Autodesk Inventor part; units mm, degrees
ref_plane "YZ Plane" through (0, 0, 0) normal (1, 0, 0) x (0, 1, 0)
ref_plane "XZ Plane" through (0, 0, 0) normal (0, 1, 0) x (-1, 0, 0)
ref_plane "XY Plane" through (0, 0, 0) normal (0, 0, 1) x (1, 0, 0)
sketch "Schizzo1" plane through (0, 0, 0) normal (0, 1, 0) x (-1, 0, 0)
  line L0 (10.5, 8) -> (-10.5, 8)
  line L1 (-10.5, 8) -> (-10.5, -8)
  line L2 (-10.5, -8) -> (10.5, -8)
  line L3 (10.5, -8) -> (10.5, 8)
  line L4 (10.5, 8) -> (-10.5, -8) construction
  line L5 (-10.5, 8) -> (10.5, -8) construction
  point P0 (0, 0)
  point P1 (0, 0)
  point P2 (0, 0)
  dimension "d0" = 16
  dimension "d1" = 21
extrude "Estrusione1" add sketch "Schizzo1" along normal blind 1.5
sketch "Schizzo2" plane through (0, 1.5, 0) normal (0, 1, 0) x (1, 0, 0)
  line L0 (10.5, 8) -> (-10.5, 8)
  line L1 (-10.5, 8) -> (-8, 8)
  line L2 (-8, 8) -> (-8, 5.5)
  line L3 (10.5, 8) -> (8, 8)
  line L4 (8, 8) -> (8, 5.5)
  point P0 (0, 0)
  dimension "d16" = 2.5
  dimension "d17" = 2.5
  dimension "d18" = 2.5
  dimension "d19" = 2.5
hole "Foro1" at (-8, 1.5, -5.5) at (8, 1.5, -5.5) direction (0, -1, 0) diameter 3.4 depth 1.5 tip angle 118
sketch "Schizzo4" plane through (0, 1.5, 0) normal (0, 1, 0) x (1, 0, 0)
  line L0 (10, -5.5) -> (-10, -5.5)
  line L1 (-10, -5.5) -> (-10, -8)
  line L2 (-10, -8) -> (10, -8)
  line L3 (10, -8) -> (10, -5.5)
  line L4 (10, -5.5) -> (-10, -8) construction
  line L5 (-10, -5.5) -> (10, -8) construction
  line L6 (-10.5, -8) -> (10.5, -8)
  point P0 (0, 0)
  point P1 (0, -6.75)
  point P2 (0, -8)
  dimension "d45" = 20
  dimension "d46" = 2.5
extrude "Estrusione2" add sketch "Schizzo4" along normal blind 2.5
sketch "Schizzo6" plane through (0, 4, 0) normal (0, 1, 0) x (1, 0, 0)
  line L0 (-8.75, -6.75) -> (-6.25, -6.75)
  line L1 (-9.05, -7.05) -> (-9.05, -6.45)
  line L2 (-9.05, -6.45) -> (-8.45, -6.45)
  line L3 (-8.45, -6.45) -> (-8.45, -7.05)
  line L4 (-8.45, -7.05) -> (-9.05, -7.05)
  line L5 (-6.25, -6.75) -> (-3.75, -6.75)
  line L6 (-6.55, -7.05) -> (-6.55, -6.45)
  line L7 (-6.55, -6.45) -> (-5.95, -6.45)
  line L8 (-5.95, -6.45) -> (-5.95, -7.05)
  line L9 (-5.95, -7.05) -> (-6.55, -7.05)
  line L10 (-3.75, -6.75) -> (-1.25, -6.75)
  line L11 (-4.05, -7.05) -> (-4.05, -6.45)
  line L12 (-4.05, -6.45) -> (-3.45, -6.45)
  line L13 (-3.45, -6.45) -> (-3.45, -7.05)
  line L14 (-3.45, -7.05) -> (-4.05, -7.05)
  line L15 (-1.25, -6.75) -> (1.25, -6.75)
  line L16 (-1.55, -7.05) -> (-1.55, -6.45)
  line L17 (-1.55, -6.45) -> (-0.95, -6.45)
  line L18 (-0.95, -6.45) -> (-0.95, -7.05)
  line L19 (-0.95, -7.05) -> (-1.55, -7.05)
  line L20 (1.25, -6.75) -> (3.75, -6.75)
  line L21 (0.95, -7.05) -> (0.95, -6.45)
  line L22 (0.95, -6.45) -> (1.55, -6.45)
  line L23 (1.55, -6.45) -> (1.55, -7.05)
  line L24 (1.55, -7.05) -> (0.95, -7.05)
  line L25 (3.75, -6.75) -> (6.25, -6.75)
  line L26 (3.45, -7.05) -> (3.45, -6.45)
  line L27 (3.45, -6.45) -> (4.05, -6.45)
  line L28 (4.05, -6.45) -> (4.05, -7.05)
  line L29 (4.05, -7.05) -> (3.45, -7.05)
  line L30 (6.25, -6.75) -> (8.75, -6.75)
  line L31 (5.95, -7.05) -> (5.95, -6.45)
  line L32 (5.95, -6.45) -> (6.55, -6.45)
  line L33 (6.55, -6.45) -> (6.55, -7.05)
  line L34 (6.55, -7.05) -> (5.95, -7.05)
  line L35 (8.45, -7.05) -> (8.45, -6.45)
  line L36 (8.45, -6.45) -> (9.05, -6.45)
  line L37 (9.05, -6.45) -> (9.05, -7.05)
  line L38 (9.05, -7.05) -> (8.45, -7.05)
  line L39 (-8.75, -6.75) -> (-10, -6.75)
  line L40 (-10, -8) -> (10, -8)
  line L41 (-10, -8) -> (-10, -6.75)
  line L42 (-10, -8) -> (-8.75, -8) construction
  point P0 (0, 0)
  dimension "d47" = 2.5
  dimension "d48" = 0.6
  dimension "d49" = 2.5
  dimension "d50" = 0.6
  dimension "d51" = 2.5
  dimension "d52" = 0.6
  dimension "d53" = 2.5
  dimension "d54" = 0.6
  dimension "d55" = 2.5
  dimension "d56" = 0.6
  dimension "d57" = 2.5
  dimension "d58" = 0.6
  dimension "d59" = 2.5
  dimension "d60" = 0.6
  dimension "d62" = 0.6
  dimension "d63" = 1.25
  dimension "d64" = 1.25
  dimension "d65" = 90
extrude "Estrusione3" add sketch "Schizzo6" along normal blind 5.75 and the other way blind 5.25
properties part number "10_MPU_6050"
Model file for the job. Use its own axes, mm. A direction names the side the tool comes from. Round coordinates to 2 decimals unless told otherwise and drop trailing zeros. Order: outer loops, then holes, each group sorted by start corner. A loop starts at its lowest first (then second) coordinate and runs counter-clockwise, first axis right, second up.
(1) Band-saw the part on D-D (x = 0.5). List the corners of the cut face in (y, z).
(2) Pin check, flat tips, straight feed: pin 1 (3 mm diameter, centred on x = 1, z = 4, fed in from -Y); pin 2 (0.5 mm diameter, centred on y = 6, z = 7, fed in from +X); pin 3 (0.5 mm diameter, centred on x = -8.5, y = 7.5, fed in from -Z); pin 4 (3 mm diameter, centred on x = 2.5, z = 6.5, fed in from +Y). Stop position of each tip, or through.
(3) Drill centre lines: line 1 (X direction, y = 0.85, z = -5.5); line 2 (Z direction, x = 8, y = 0.6); line 3 (Y direction, x = 1.75, z = 6.25). Where is each one in solid material? Low to high.
(4) Pull direction X, two halves, no side cores. Call faces 6 (the face through (10.5, 1, 0)), 7 (the face through (0, 4, 7)), 8 (the face through (0, 1, -8)), 9 (the face through (-9.686, 0.74, -5.721)): released by +X, released by -X, zero draft, split by the parting line, or undercut.
(5) Band-saw the part on A-A (z = -5.5). List the corners of the cut face in (x, y), then the cut area to 3 significant figures.
(6) Band-saw the part on C-C (x = 8). List the corners of the cut face in (y, z), then the cut area to 4 significant figures.
(7) Band-saw the part on B-B (y = 5.5). Give the number of separate pieces and of enclosed holes in the cut face, then the cut area to 3 significant figures.
(8) 3-axis set-ups, long thin cutter, end or side, ignore diameter. For faces 1 (the face through (9.66, 0.74, -5.87)), 2 (the face through (0, 3, 5.5)), 3 (the face through (-10.5, 1, 0)), 4 (the face through (-10, 3, 7)), 5 (the face through (10, 3, 7)): which of +Z, -Z, +X, -X, +Y, -Y reach the whole face in a straight line?
Verdict:
1. outline: (0, -8) - (1.5, -8) - (1.5, 5.5) - (4, 5.5) - (4, 8) - (0, 8) - close
2. pin 1: stops at y = 0
2. pin 2: stops at x = 9.05
2. pin 3: stops at z = 6.45
2. pin 4: stops at y = 9.75
3. line 1: x = -10.5 to -9.7, -6.3 to 6.3, 9.7 to 10.5
3. line 2: z = -8 to -7.2, -3.8 to 8
3. line 3: y = 0 to 4
4. face 6: released by +X
4. face 7: undercut
4. face 8: zero draft
4. face 9: undercut
5. outline: (-10.5, 0) - (-9.7, 0) - (-9.7, 1.5) - (-10.5, 1.5) - close; (-6.3, 0) - (6.3, 0) - (6.3, 1.5) - (-6.3, 1.5) - close; (9.7, 0) - (10.5, 0) - (10.5, 1.5) - (9.7, 1.5) - close
5. area: 21.3 mm2
6. outline: (0, -8) - (1.5, -8) - (1.5, -7.2) - (0, -7.2) - close; (0, -3.8) - (1.5, -3.8) - (1.5, 5.5) - (4, 5.5) - (4, 8) - (0, 8) - close
6. area: 25.15 mm2
7. separate pieces: 8
7. enclosed holes: 0
7. area: 2.88 mm2
8. face 1: +Y, -Y
8. face 2: -Z, +X, -X, +Y
8. face 3: +Z, -Z, -X, +Y, -Y
8. face 4: +Z, -Z, -X, +Y
8. face 5: +Z, -Z, +X, +Y
